```python
from build123d import *
from OCP.BRepFilletAPI import BRepFilletAPI_MakeChamfer

# Parameters (mm, degrees)
SKETCH1_W           = 45
SKETCH1_H           = 26
BOSS_EXTRUDE1_DEPTH = 13.5
SKETCH2_W           = 47
SKETCH2_H           = 28
SKETCH2_W_2         = 35
SKETCH2_H_2         = 16
BOSS_EXTRUDE2_DEPTH = 2
CHAMFER1_SIZE       = 2
CHAMFER1_SIZE_2     = 1.154700538
CUT_EXTRUDE1_DEPTH  = 13.5


with BuildPart() as part:
    # Sketch1 → Boss-Extrude1 (new body)
    with BuildSketch(Plane(origin=(0, 0, 0), x_dir=(1, 0, 0), z_dir=(0, 1, 0))):
        Rectangle(SKETCH1_W, SKETCH1_H)
    extrude(amount=BOSS_EXTRUDE1_DEPTH)

    # Sketch2 → Boss-Extrude2 (add)
    with BuildSketch(Plane(origin=(0, 13.5, 0), x_dir=(1, 0, 0), z_dir=(0, 1, 0))):
        Rectangle(SKETCH2_W, SKETCH2_H)
        Rectangle(SKETCH2_W_2, SKETCH2_H_2, mode=Mode.SUBTRACT)
    extrude(amount=BOSS_EXTRUDE2_DEPTH)

    # Chamfer1
    chamfer1_edges_1 = [part.edges().sort_by_distance(p)[0] for p in [
        (0, 15.5, -8),
    ]]
    chamfer1_side_1 = [part.faces().sort_by_distance(p)[0] for p in [
        (0, 15.5, -8.023094011),
    ]]
    chamfer1_edges_2 = [part.edges().sort_by_distance(p)[0] for p in [
        (-17.5, 15.5, 0),
    ]]
    chamfer1_side_2 = [part.faces().sort_by_distance(p)[0] for p in [
        (-17.523094011, 15.5, 0),
    ]]
    chamfer1_edges_3 = [part.edges().sort_by_distance(p)[0] for p in [
        (0, 15.5, 8),
    ]]
    chamfer1_side_3 = [part.faces().sort_by_distance(p)[0] for p in [
        (0, 15.5, 8.023094011),
    ]]
    chamfer1_edges_4 = [part.edges().sort_by_distance(p)[0] for p in [
        (17.5, 15.5, 0),
    ]]
    chamfer1_side_4 = [part.faces().sort_by_distance(p)[0] for p in [
        (17.523094011, 15.5, 0),
    ]]
    chamfer1_edges_5 = [part.edges().sort_by_distance(p)[0] for p in [
        (-23.5, 15.5, 0),
    ]]
    chamfer1_side_5 = [part.faces().sort_by_distance(p)[0] for p in [
        (-23.5, 15.476905989, 0),
    ]]
    chamfer1_edges_6 = [part.edges().sort_by_distance(p)[0] for p in [
        (0, 15.5, -14),
    ]]
    chamfer1_side_6 = [part.faces().sort_by_distance(p)[0] for p in [
        (0, 15.476905989, -14),
    ]]
    chamfer1_edges_7 = [part.edges().sort_by_distance(p)[0] for p in [
        (23.5, 15.5, 0),
    ]]
    chamfer1_side_7 = [part.faces().sort_by_distance(p)[0] for p in [
        (23.5, 15.476905989, 0),
    ]]
    chamfer1_edges_8 = [part.edges().sort_by_distance(p)[0] for p in [
        (0, 15.5, 14),
    ]]
    chamfer1_side_8 = [part.faces().sort_by_distance(p)[0] for p in [
        (0, 15.476905989, 14),
    ]]
    chamfer1 = BRepFilletAPI_MakeChamfer(part.part.solid().wrapped)
    for e in chamfer1_edges_1:
        chamfer1.Add(CHAMFER1_SIZE - 0.0001, CHAMFER1_SIZE_2 - 0.0001, e.wrapped, chamfer1_side_1[0].wrapped)
    for e in chamfer1_edges_2:
        chamfer1.Add(CHAMFER1_SIZE - 0.0001, CHAMFER1_SIZE_2 - 0.0001, e.wrapped, chamfer1_side_2[0].wrapped)
    for e in chamfer1_edges_3:
        chamfer1.Add(CHAMFER1_SIZE - 0.0001, CHAMFER1_SIZE_2 - 0.0001, e.wrapped, chamfer1_side_3[0].wrapped)
    for e in chamfer1_edges_4:
        chamfer1.Add(CHAMFER1_SIZE - 0.0001, CHAMFER1_SIZE_2 - 0.0001, e.wrapped, chamfer1_side_4[0].wrapped)
    for e in chamfer1_edges_5:
        chamfer1.Add(CHAMFER1_SIZE - 0.0001, CHAMFER1_SIZE_2 - 0.0001, e.wrapped, chamfer1_side_5[0].wrapped)
    for e in chamfer1_edges_6:
        chamfer1.Add(CHAMFER1_SIZE - 0.0001, CHAMFER1_SIZE_2 - 0.0001, e.wrapped, chamfer1_side_6[0].wrapped)
    for e in chamfer1_edges_7:
        chamfer1.Add(CHAMFER1_SIZE - 0.0001, CHAMFER1_SIZE_2 - 0.0001, e.wrapped, chamfer1_side_7[0].wrapped)
    for e in chamfer1_edges_8:
        chamfer1.Add(CHAMFER1_SIZE - 0.0001, CHAMFER1_SIZE_2 - 0.0001, e.wrapped, chamfer1_side_8[0].wrapped)
    add(Compound.cast(chamfer1.Shape()), mode=Mode.REPLACE)  # a hair under: the kernel refuses the full size

    # Sketch3 → Cut-Extrude1 (cut)
    with BuildSketch(Plane.XZ):
        with BuildLine():
            Line((-22, -4), (-19.5, -4))
            ThreePointArc((-19.5, -4), (-18, -5.5), (-19.5, -7))
            Line((-19.5, -7), (-22, -7))
            Line((-22, -7), (-22, -4))
        make_face()
    extrude(amount=-CUT_EXTRUDE1_DEPTH, mode=Mode.SUBTRACT)


solid = part.part
```
Check sheet for the modelled part. Datum: model origin and axes. Units: mm. A direction names the side the tool comes from. Round coordinates to 2 decimals unless told otherwise and drop trailing zeros. Write each loop counter-clockwise with the first axis right and the second up, starting at its lowest first coordinate (ties: lowest second). Pieces come first, ordered by that corner, then holes. Notation, with made-up numbers: (15.5, -9.75) -> (20.5, -9.75) arc R10 cw to (20.5, 7.25) -> close; hole circle Ø8 at (-7, 32). An arc over 180 degrees is marked (long way). Put each result on its own line as item: value.
(1) Mould release check, pull along X, two halves, no side actions. Record for faces 1 (the face through (-21, 7, -7)), 2 (the face through (-0.273, 14.915, 8.986)), 3 (the face through (-0.329, 14.514, 13.415)), 4 (the face through (22.915, 14.514, 0.196)): released by +X, released by -X, zero draft, split by the parting line, or undercut.
Values found:
face 1: undercut
face 2: undercut
face 3: zero draft
face 4: released by +X
(2) Tool access check on faces 5 (the face through (22.5, 7, 0)), 6 (the face through (0, 13.5, 0)), 7 (the face through (-18, 6.7, -5.5)). Record the directions out of +Z, -Z, +X, -X, +Y, -Y that give a thin tool (end or side, any length) a straight path to the whole face; none if there is none.
Values found:
face 5: +Z, -Z, +X, -Y
face 6: +Y
face 7: -Y
(3) Material ranges on line 1 (X direction, y = 13, z = -0.5); line 2 (Z direction, x = -1.5, y = 9.75); line 3 (Y direction, x = -14.5, z = 7.5), recorded low to high.
Values found:
line 1: x = -22.5 to 22.5
line 2: z = -13 to 13
line 3: y = 0 to 13.5
(4) Go/stop test with flat-tipped pins: pin 1 Ø2.5 at (y, z) = (8.5, -6) entering from +X; pin 2 Ø4 at (x, y) = (-9.5, 5.5) entering from +Z; pin 3 Ø0.9 at (x, z) = (-20, -5.5) entering from -Y. Record where each tip stops, or that it passes through.
Values found:
pin 1: stops at x = 22.5
pin 2: stops at z = 13
pin 3: stops at y = 13.5
(5) Sectioned sample at A-A (y = 10.5). Enter the section's corners in (x, z).
Values found:
outline: (-22.5, -13) -> (22.5, -13) -> (22.5, 13) -> (-22.5, 13) -> close; hole (-22, -7) -> (-19.5, -7) arc R1.5 ccw to (-19.5, -4) -> (-22, -4) -> close
